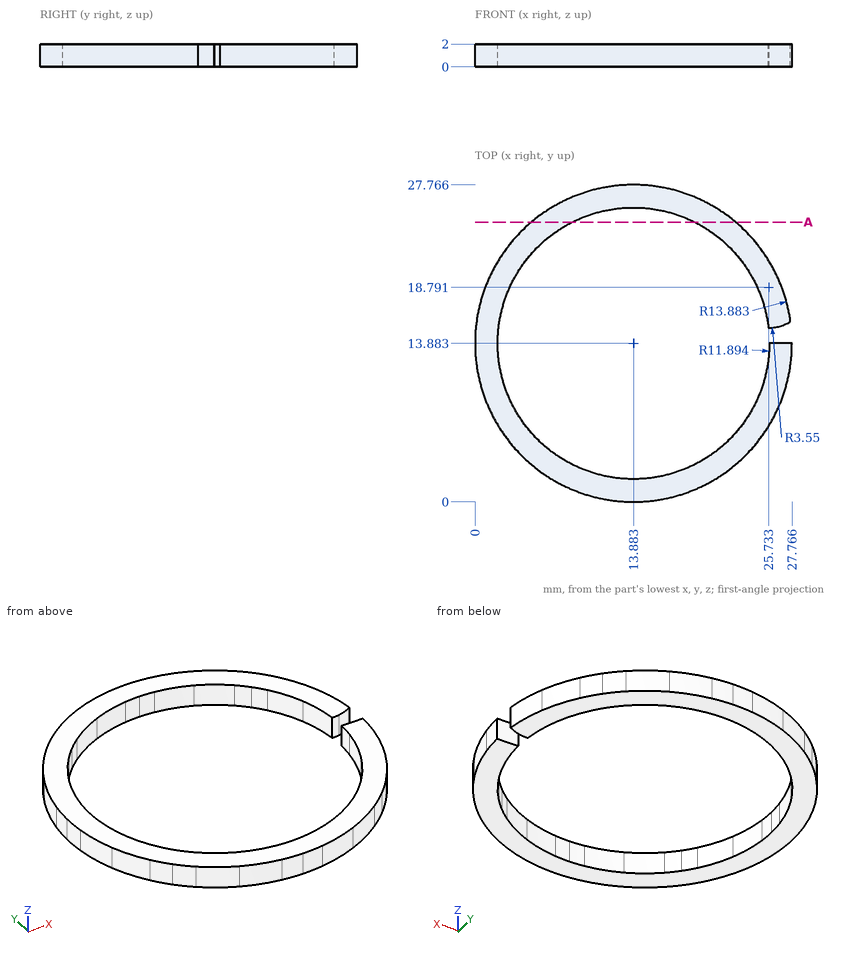
For this review, use the dimensioned drawing (mm, ordinates from the lowest corner) and the shaded views. Round coordinates to 2 decimals unless told otherwise and drop trailing zeros. Order: outer loops, then holes, each group sorted by start corner. A loop starts at its lowest first (then second) coordinate and runs counter-clockwise, first axis right, second up. Notation, with made-up numbers: (9, -27.5) -> (49, -27.5) arc R9 ccw to (49, -22.5) -> close; hole circle Ø5 at (-30.75, -17.75). An arc over 180 degrees is marked (long way). One line per item, written item: value. Start each with the question number.
Q1. Clearance check with flat-ended pins moving along their axes: pin 1 Ø1 at (x, z) = (26.5, 1.5) entering from +Y; pin 2 Ø5 at (x, y) = (10.5, 22.5) entering from -Z; pin 3 Ø1 at (y, z) = (4.5, 0.5) entering from -X (1 decimal); pin 4 Ø1 at (y, z) = (20, 1.5) entering from -X. State where each tip first meets the part, or that it passes through.
Q2. Take a section at A-A (y = 24.5). Write out the cut boundary in (x, z).
Q3. Wall thickness on line 1 (X direction, y = 9.75, z = 0.85) (1 decimal); line 2 (X direction, y = 10.75, z = 0.95); line 3 (Y direction, x = 20.25, z = 0.1) (1 decimal): over which ranges is each line inside the solid? List them lowest first.
Reported:
1. pin 1: stops at y = 20.66
1. pin 2: passes through
1. pin 3: stops at x = 3.2
1. pin 4: stops at x = 1.19
2. outline: (4.94, 0) -> (8.52, 0) -> (8.52, 2) -> (4.94, 2) -> close; (19.24, 0) -> (22.83, 0) -> (22.83, 2) -> (19.24, 2) -> close
3. line 1: x = 0.6 to 2.7, 25 to 27.1
3. line 2: x = 0.36 to 2.41, 25.36 to 27.41
3. line 3: y = 1.5 to 3.8, 23.9 to 26.2
